For this review, take the finished solid that the model builds, in its own axes (mm). A direction names the side the tool comes from. Coordinates: 2 decimals unless noted, no trailing zeros. Write each loop counter-clockwise with the first axis right and the second up, starting at its lowest first coordinate (ties: lowest second). Pieces come first, ordered by that corner, then holes. Notation, with made-up numbers: (6, -38.5) -> (28, -38.5) arc R21 cw to (28, -21.5) -> close; hole circle Ø1 at (89, 15). An arc over 180 degrees is marked (long way). One line per item, written item: value. Start each with the question number.
1) Mouldability with a two-part tool opening along X and no side actions: class faces 1 (the flat face through (-37, 3, -25.4)), 2 (the cylindrical face through (34.906, 3.131, 1.138)), 3 (the flat face through (4.342, 6.439, -4.634)) as released by +X, released by -X, zero draft, split by the parting line, or undercut.
2) Add section A-A (y = 9.75). State the section outline as (x, z) points (3 decimals).
3) For pin 1 Ø3 at (y, z) = (5.5, -26) entering from -X; pin 2 Ø4 at (x, y) = (-18.5, 5.5) entering from -Z; pin 3 Ø4 at (x, y) = (-25, 7.5) entering from -Z; pin 4 Ø1.9 at (x, y) = (-39.5, 2.5) entering from -Z, all flat-tipped, find the tip position at first contact; note any pin that passes through.
4) Add section D-D (z = -13.5). State the section outline as (x, y) points.
5) Add section B-B (x = -3). State the section outline as (y, z) points, and give its area (3 significant figures).
6) Machinability: for faces 4 (the flat face through (-1.842, 6.439, -6.077)), 5 (the cylindrical face through (-15.497, 9.481, -3.441)), 6 (the flat face through (-8, 0, 0)), 7 (the flat face through (-37, 3, 25.4)), 8 (the flat face through (-7, 12.7, 0)), which of the approach directions +Z, -Z, +X, -X, +Y, -Y give a long, thin tool a straight path to every point of the face, cutting with its end or side? Answer none if there is none.
7) For probe 1 along Z at (x, y) = (-30.5, 4.75); probe 2 along Y at (x, z) = (22, 5.5); probe 3 along Z at (x, y) = (3.5, 3.25), list the stretches that pass through material, from the lowest coordinate up. Write a range as from..to.
from build123d import *

# Parameters (mm, degrees)
SKETCH1_R           = 34.925
SKETCH1_W           = 25.4
SKETCH1_H           = 50.8
BOSS_EXTRUDE1_DEPTH = 6.35
SKETCH2_R           = 15.875
BOSS_EXTRUDE2_DEPTH = 6.35
CUT_EXTRUDE1_DEPTH  = 62.794126307


with BuildPart() as part:
    # Sketch1 → Boss-Extrude1 (new body)
    with BuildSketch(Plane(origin=(0, 0, 0), x_dir=(1, 0, 0), z_dir=(0, 1, 0))):
        Circle(SKETCH1_R)
        with Locations((-36.670724332, 0)):
            Rectangle(SKETCH1_W, SKETCH1_H)
    extrude(amount=BOSS_EXTRUDE1_DEPTH)

    # Sketch2 → Boss-Extrude2 (add)
    with BuildSketch(Plane(origin=(0, 6.35, 0), x_dir=(1, 0, 0), z_dir=(0, 1, 0))):
        with Locations(Location((0, 0, 0), (0, 0, 270))):
            Circle(SKETCH2_R)
    extrude(amount=BOSS_EXTRUDE2_DEPTH)

    # Sketch3 → Cut-Extrude1 (cut, through all)
    with BuildSketch(Plane(origin=(0, 12.7, 0), x_dir=(1, 0, 0), z_dir=(0, 1, 0))):
        Polygon((5.391213117, -4.969723781), (6.999513603, 2.184065626), (1.608300486, 7.153789407), (-5.391213117, 4.969723781), (-6.999513603, -2.184065626), (-1.608300486, -7.153789407), align=None)
    extrude(amount=-CUT_EXTRUDE1_DEPTH, mode=Mode.SUBTRACT)


solid = part.part
Numbers:
1. face 1: zero draft
1. face 2: split by the parting line
1. face 3: undercut
2. outline: circle Ø31.75 at (0, 0); hole (-7, 2.184) -> (-5.391, -4.97) -> (1.608, -7.154) -> (7, -2.184) -> (5.391, 4.97) -> (-1.608, 7.154) -> close
3. pin 1: x = -49.37
3. pin 2: z = -30.78
3. pin 3: z = -25.96
3. pin 4: z = -25.4
4. outline: (-49.37, 0) -> (32.21, 0) -> (32.21, 6.35) -> (8.35, 6.35) -> (8.35, 12.7) -> (-8.35, 12.7) -> (-8.35, 6.35) -> (-49.37, 6.35) -> close
5. outline: (0, -34.8) -> (6.35, -34.8) -> (6.35, -15.59) -> (12.7, -15.59) -> (12.7, -5.72) -> (0, -5.72) -> close; (0, 5.87) -> (12.7, 5.87) -> (12.7, 15.59) -> (6.35, 15.59) -> (6.35, 34.8) -> (0, 34.8) -> close
5. area: 493 mm²
6. face 4: +Y, -Y
6. face 5: +Y
6. face 6: +Z, -Z, +X, -X, -Y
6. face 7: +Z, -X, +Y, -Y
6. face 8: +Z, -Z, +X, -X, +Y
7. probe 1: -25.4..25.4
7. probe 2: 0..6.35
7. probe 3: -34.75..-5.41, 5.56..34.75
